```python
from build123d import *

# Parameters (mm, degrees)
F0_W     = 31.75
F0_H     = 15.875
F0_R     = 2.38125
F1_DEPTH = 3.175
F2_DEPTH = 4.7625
F3_T     = -1.5875
F4_R     = 3.175
F4_R_2   = 2.38125
F5_DEPTH = 1.5875


with BuildPart() as f1:
    # F0 (on Top) → F1 (new body)
    with BuildSketch(Plane.XY):
        Rectangle(F0_W, F0_H)
        with Locations((-11.90625, -3.96875)):
            Circle(F0_R, mode=Mode.SUBTRACT)
        with Locations((-3.96875, -3.96875)):
            Circle(F0_R, mode=Mode.SUBTRACT)
        with Locations((3.96875, -3.96875)):
            Circle(F0_R, mode=Mode.SUBTRACT)
        with Locations((11.90625, -3.96875)):
            Circle(F0_R, mode=Mode.SUBTRACT)
        with Locations((-11.90625, 3.96875)):
            Circle(F0_R, mode=Mode.SUBTRACT)
        with Locations((-3.96875, 3.96875)):
            Circle(F0_R, mode=Mode.SUBTRACT)
        with Locations((3.96875, 3.96875)):
            Circle(F0_R, mode=Mode.SUBTRACT)
        with Locations((11.90625, 3.96875)):
            Circle(F0_R, mode=Mode.SUBTRACT)
    extrude(amount=F1_DEPTH)

    # F0 (on Top) → F2 (join)
    with BuildSketch(Plane.XY):
        with Locations((-11.90625, 3.96875)):
            Circle(F0_R)
        with Locations((-3.96875, 3.96875)):
            Circle(F0_R)
        with Locations((-3.96875, -3.96875)):
            Circle(F0_R)
        with Locations((-11.90625, -3.96875)):
            Circle(F0_R)
        with Locations((3.96875, 3.96875)):
            Circle(F0_R)
        with Locations((11.90625, 3.96875)):
            Circle(F0_R)
        with Locations((11.90625, -3.96875)):
            Circle(F0_R)
        with Locations((3.96875, -3.96875)):
            Circle(F0_R)
    extrude(amount=F2_DEPTH)

    # F3
    f3_openings = [f1.faces().sort_by_distance(p)[0] for p in [
        (0, 0, 0),
    ]]
    offset(amount=F3_T, openings=f3_openings, kind=Kind.INTERSECTION)

    # F4 (on face) → F5 (join)
    with BuildSketch(Plane(origin=(0, 0, 1.5875), x_dir=(1, 0, 0), z_dir=(0, 0, -1))):
        Circle(F4_R)
        Circle(F4_R_2, mode=Mode.SUBTRACT)
    extrude(amount=F5_DEPTH)


solid = f1.part
```
The listing builds one solid part. Answer for the finished solid, in the listing's coordinates (mm). A direction names the side the tool comes from. Coordinates: 2 decimals unless noted, no trailing zeros. Loops run counter-clockwise (first coordinate to the right, second up) from the corner with the lowest first, then second, coordinate; pieces in that order, holes last. Notation, with made-up numbers: M 38.5,36 L 72.5,36 A20 ccw 72.5,56 Z; hole C 81.25,78 d1. An arc over 180 degrees is marked long. Answer as CSV lines item,"result". Start each with the question number.
(1) The part is cut by section C-C (y = 0). Give the vertices of the cut face in (x, z) (1 decimal).
(2) Given pin 1 (0.8 mm diameter, centred on x = 12, y = 3.5, fed in from -Z); pin 2 (0.8 mm diameter, centred on x = 4, y = 4, fed in from -Z) (3 decimals); pin 3 (4 mm diameter, centred on x = 0, y = 0, fed in from +Z) (3 decimals), each flat-ended and moving along its own axis, determine where each tip first touches the part or whether it passes through.
(3) The part is cut by section A-A (z = 0.4). State how many separate pieces and enclosed holes the cut face has, and give its area (3 significant figures).
(4) For faces 3 (the cylindrical face through (-1.697, 4.684, 3.958)), 4 (the flat face through (-12, 4, 4.762)), 5 (the flat face through (-4, 4, 3.175)), determine the directions among +Z, -Z, +X, -X, +Y, -Y from which every point of the face is accessible in a straight line to the end or side of a thin tool.
(5) The mould has two halves that part along Y. Classify faces 1 (the flat face through (0, 7, 0)), 2 (the cylindrical face through (4.726, 4.207, 2.37)): pulls with the +Y half, pulls with the -Y half, needs draft (parallel to the pull), parting line crosses it, or undercut.
(6) Find the intervals of material crossed by L1, parallel to Y at x = 4, z = 1.2; L2, parallel to X at y = 5, z = 0.9 (1 decimal), in increasing order. Write a range as [from, to].
Determined:
1,outline,"M -15.9,0 L -14.3,0 L -14.3,1.6 L -3.2,1.6 L -3.2,0 L -2.4,0 L -2.4,1.6 L 2.4,1.6 L 2.4,0 L 3.2,0 L 3.2,1.6 L 14.3,1.6 L 14.3,0 L 15.9,0 L 15.9,3.2 L -15.9,3.2 Z"
2,pin 1,"z = 1.59"
2,pin 2,"z = 3.175"
2,pin 3,"z = 3.175"
3,separate pieces,"2"
3,enclosed holes,"2"
3,area,"155 mm2"
4,face 3,"+Z"
4,face 4,"+Z, +X, -X, +Y, -Y"
4,face 5,"-Z"
5,face 1,"needs draft"
5,face 2,"undercut"
6,L1,"[-7.94, -6.35], [6.35, 7.94]"
6,L2,"[-15.9, -14.3], [14.3, 15.9]"
